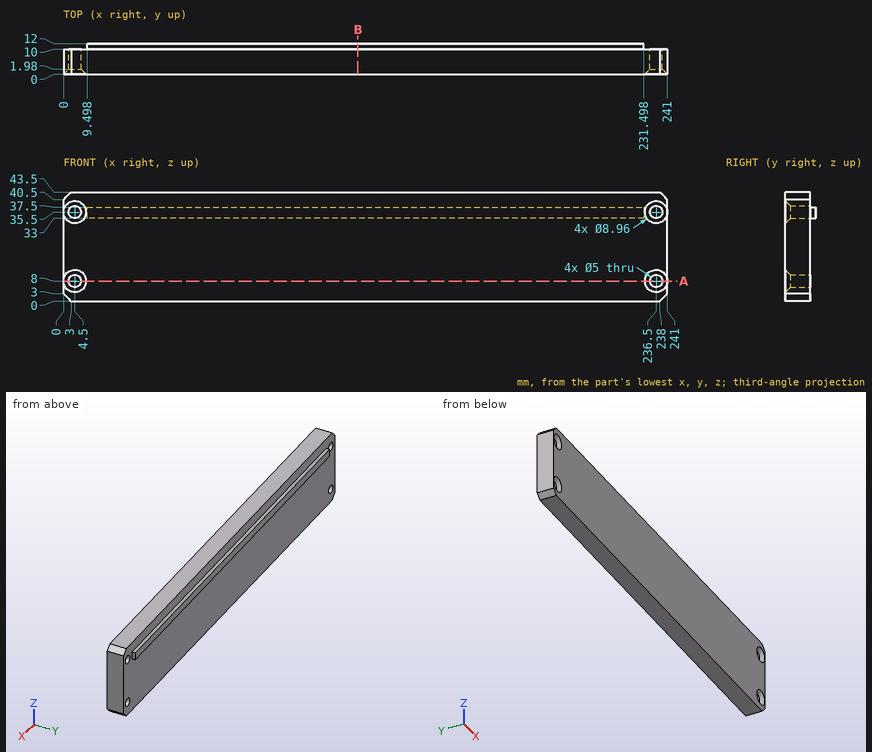
For this review, use the dimensioned drawing (mm, ordinates from the lowest corner) and the shaded views. Round coordinates to 2 decimals unless told otherwise and drop trailing zeros. Order: outer loops, then holes, each group sorted by start corner. A loop starts at its lowest first (then second) coordinate and runs counter-clockwise, first axis right, second up.
1) Consider section B-B (x = 117.5). State the section outline as (y, z) points, plus the area to 3 significant figures.
The answers:
outline: (0, 0) - (10, 0) - (10, 33) - (12, 33) - (12, 37.5) - (10, 37.5) - (10, 43.5) - (0, 43.5) - close
area: 444 mm2
2) For L1, parallel to Z at x = 4.5, y = 6; L2, parallel to X at y = 4.75, z = 8; L3, parallel to X at y = 4.75, z = 10, list the stretches that pass through material, from the lowest coordinate up.
The answers:
L1: z = 0 to 5.5, 10.5 to 33, 38 to 43.5
L2: x = 0 to 2, 7 to 234, 239 to 241
L3: x = 0 to 3, 6 to 235, 238 to 241
3) Clearance check with flat-ended pins moving along their axes: pin 1 Ø1 at (x, y) = (131, 11.5) entering from +Z; pin 2 Ø1.6 at (y, z) = (11, 34) entering from +X; pin 3 Ø8 at (x, z) = (156, 13.5) entering from +Y. State where each tip first meets the part, or that it passes through.
The answers:
pin 1: stops at z = 37.5
pin 2: stops at x = 231.5
pin 3: stops at y = 10
4) Consider section A-A (z = 8). Count the separate pieces of the cut face and the enclosed holes in it, plus the area to 3 significant figures.
The answers:
separate pieces: 3
enclosed holes: 0
area: 2,300 mm2
